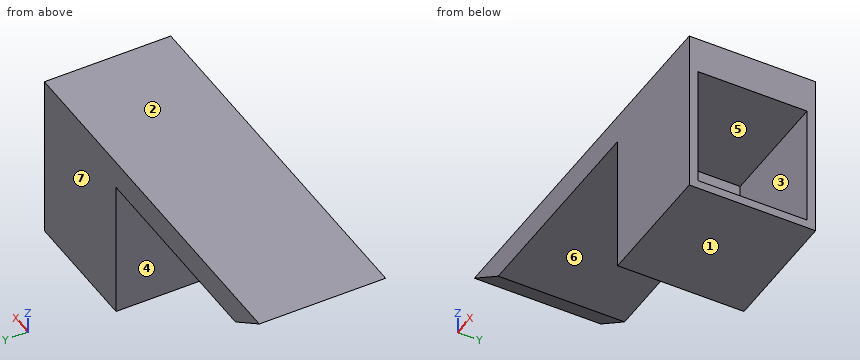
from build123d import *

# Parameters (mm, degrees)
F0_W     = 1500
F0_H     = 750
F1_DEPTH = 1000
F3_DEPTH = 750
F4_DEPTH = 750
F6_DEPTH = 750
F8_W     = 648.4
F8_H     = 731.364360714
F9_DEPTH = 700


with BuildPart() as f1:
    # F0 (on Top) → F1 (new body)
    with BuildSketch(Plane.XY):
        Rectangle(F0_W, F0_H)
    extrude(amount=-F1_DEPTH)

    # F2 (on face) → F3 (cut)
    with BuildSketch(Plane.XZ.offset(375)):
        Polygon((-750, -1000), (750, -1000), (-750, 0), align=None)
    extrude(amount=-F3_DEPTH, mode=Mode.SUBTRACT)

    # F4 (add): a face of the model
    f4_faces = [f1.faces().sort_by_distance(p)[0] for p in [
        (750, 0, -500),
    ]]
    extrude(f4_faces, amount=F4_DEPTH)

    # F5 (on face) → F6 (cut)
    with BuildSketch(Plane.XZ.offset(375)):
        Polygon((750, -166.4100588676), (-500.3849116986, -166.4100588676), (750, -1000), align=None)
        Polygon((750, -1000), (-500.3849116986, -166.4100588676), (-500.3849116986, -1000), align=None)
    extrude(amount=-F6_DEPTH, mode=Mode.SUBTRACT)

    # F8 (on face) → F9 (cut)
    with BuildSketch(Plane.YZ.offset(1500)):
        with Locations((0, -583.517819643)):
            Rectangle(F8_W, F8_H)
    extrude(amount=-F9_DEPTH, mode=Mode.SUBTRACT)


solid = f1.part
Verification items for the finished model (mm, model axes). Face numbers are marked on the shaded views. A direction names the side the tool comes from. Coordinates: 2 decimals unless noted, no trailing zeros. Write each loop counter-clockwise with the first axis right and the second up, starting at its lowest first coordinate (ties: lowest second). Pieces come first, ordered by that corner, then holes. Notation, with made-up numbers: M 72.25,87 L 85.25,87 A8 cw 85.25,94 Z; hole C 50,65 d9. An arc over 180 degrees is marked long. Use a Markdown table: item, result.
Q1. Sectioned sample at C-C, the plane z = -667. Record the boundary of the cut face in (x, y).
Reply:
| item | result |
|---|---|
| outline | M 750,-375 L 1500,-375 L 1500,-324.2 L 800,-324.2 L 800,324.2 L 1500,324.2 L 1500,375 L 750,375 Z |
Q2. Go/stop test with flat-tipped pins: P1, Ø6, axis at y = 78, z = -281.5, coming from the -X side; P2, Ø10, axis at x = 544.5, y = 155, coming from the -Z side; P3, Ø3, axis at y = -132.5, z = -446.5, coming from the +X side. Record where each tip stops, or that it passes through.
Reply:
| item | result |
|---|---|
| P1 | stops at x = 750 |
| P2 | stops at z = -166.41 |
| P3 | stops at x = 800 |
Q3. Set-up check for the marked faces 5, 6 and 7: record each of +Z, -Z, +X, -X, +Y, -Y from which the full face is reachable in a straight line by a thin tool's end or side.
Reply:
| item | result |
|---|---|
| face 5 | +X |
| face 6 | -Z, -X, +Y, -Y |
| face 7 | +Z, -Z, +X, -X, +Y |
Q4. Thickness scan on line 1 (Y direction, x = 1224.5, z = -680); line 2 (Z direction, x = 1262, y = 55); line 3 (X direction, y = -34.5, z = -906). Record the ranges inside material, lowest first.
Reply:
| item | result |
|---|---|
| line 1 | y = -375 to -324.2, 324.2 to 375 |
| line 2 | z = -1000 to -949.2, -217.84 to 0 |
| line 3 | x = 750 to 800 |
Q5. Draft check along Z on the marked faces 1, 2, 3 and 4. Enter one of: +Z half, -Z half, draft (parallel to the pull), parting line (faces both ways), or undercut.
Reply:
| item | result |
|---|---|
| face 1 | -Z half |
| face 2 | +Z half |
| face 3 | undercut |
| face 4 | draft |
Q6. Sectioned sample at A-A, the plane x = 878. Record the boundary of the cut face in (y, z), plus the area to 3 significant figures.
Reply:
| item | result |
|---|---|
| outline | M -375,-1000 L 375,-1000 L 375,0 L -375,0 Z; hole M -324.2,-949.2 L 324.2,-949.2 L 324.2,-217.84 L -324.2,-217.84 Z |
| area | 276,000 mm² |
Q7. Sectioned sample at B-B, the plane y = -254.5. Record the boundary of the cut face in (x, z).
Reply:
| item | result |
|---|---|
| outline | M -750,0 L -500.38,-166.41 L 750,-166.41 L 750,-1000 L 1500,-1000 L 1500,-949.2 L 800,-949.2 L 800,-217.84 L 1500,-217.84 L 1500,0 Z |
Q8. Sectioned sample at D-D, the plane x = 77. Record the boundary of the cut face in (y, z), plus the area to 3 significant figures.
Reply:
| item | result |
|---|---|
| outline | M -375,-166.41 L 375,-166.41 L 375,0 L -375,0 Z |
| area | 125,000 mm² |
